Here's the drawing with two shaded views (mm, measured from the low corner). I have some questions. Round coordinates to 2 decimals unless told otherwise and drop trailing zeros. Loops run counter-clockwise (first coordinate to the right, second up) from the corner with the lowest first, then second, coordinate; pieces in that order, holes last. Notation, with made-up numbers: (72, 7) - (89, 7) arc R23 cw to (89, 34) - close; hole circle Ø8 at (-3, 52.5). An arc over 180 degrees is marked (long way). Use one line per item in the form item = value.
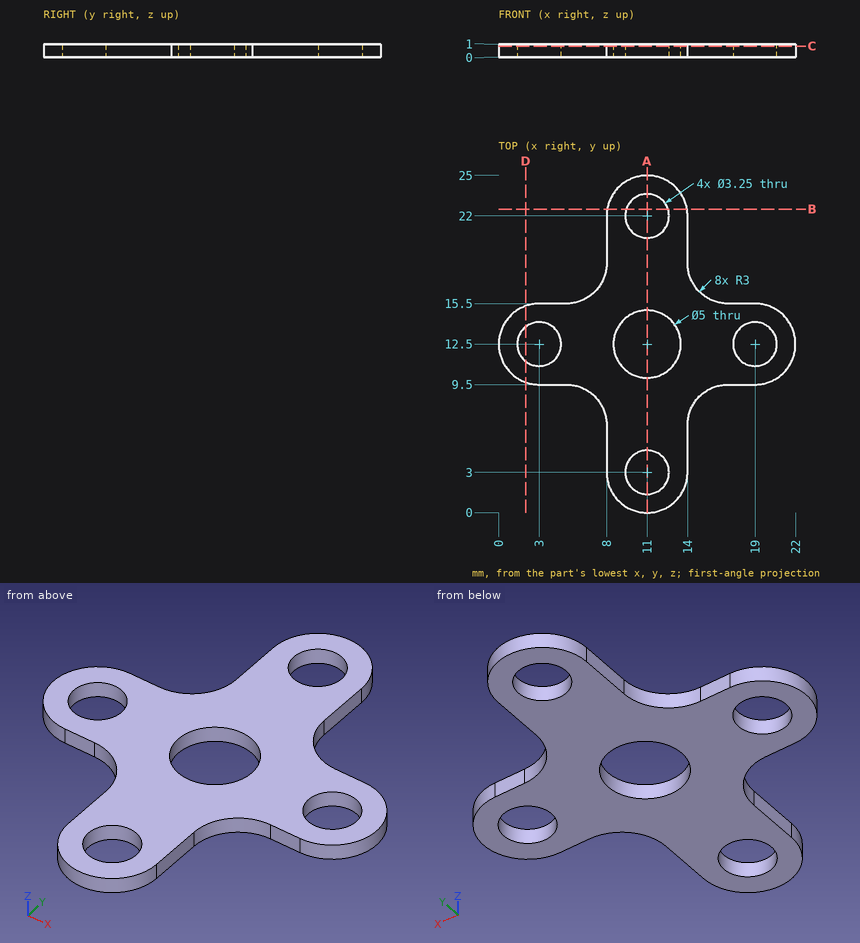
1. If we section it at A-A, the plane x = 11: Write out the boundary of the cut face in (y, z) (3 decimals), plus the area to 3 significant figures.
Solution:
outline = (0, 0) - (1.375, 0) - (1.375, 1) - (0, 1) - close; (4.625, 0) - (10, 0) - (10, 1) - (4.625, 1) - close; (15, 0) - (20.375, 0) - (20.375, 1) - (15, 1) - close; (23.625, 0) - (25, 0) - (25, 1) - (23.625, 1) - close
area = 13.5 mm^2
2. If we section it at B-B, the plane y = 22.5: Write out the boundary of the cut face in (x, z).
Solution:
outline = (8.04, 0) - (9.45, 0) - (9.45, 1) - (8.04, 1) - close; (12.55, 0) - (13.96, 0) - (13.96, 1) - (12.55, 1) - close
3. For P1, Ø5, axis at x = 11, y = 22, coming from the -Z side; P2, Ø3, axis at x = 19, y = 12.5, coming from the -Z side; P3, Ø0.5, axis at y = 5, z = 0.5, coming from the -X side; P4, Ø0.5, axis at x = 17.5, z = 0.5, coming from the +Y side, each with a flat end and sliding along its axis, tell me the tip position at first contact or that it passes through.
Solution:
P1 = 0
P2 = through
P3 = 8
P4 = 15.5
4. Please list where these lines run through material, in increasing order: line 1 along Y through (x, z) = (11, 0.55) (3 decimals); line 2 along Y through (x, z) = (3, 0.7) (3 decimals); line 3 along X through (y, z) = (20, 0.35).
Solution:
line_1 = 0 to 1.375, 4.625 to 10, 15 to 20.375, 23.625 to 25
line_2 = 9.5 to 10.875, 14.125 to 15.5
line_3 = 8 to 14
5. If we section it at C-C, the plane z = 0.85: Write out the boundary of the cut face in (x, y) (3 decimals).
Solution:
outline = (3, 9.5) - (5, 9.5) arc R3 cw to (8, 6.5) - (8, 3) arc R3 ccw to (14, 3) - (14, 6.5) arc R3 cw to (17, 9.5) - (19, 9.5) arc R3 ccw to (19, 15.5) - (17, 15.5) arc R3 cw to (14, 18.5) - (14, 22) arc R3 ccw to (8, 22) - (8, 18.5) arc R3 cw to (5, 15.5) - (3, 15.5) arc R3 ccw to start; hole circle Ø3.25 at (3, 12.5); hole circle Ø5 at (11, 12.5); hole circle Ø3.25 at (11, 3); hole circle Ø3.25 at (11, 22); hole circle Ø3.25 at (19, 12.5)
6. If we section it at D-D, the plane x = 2: Write out the boundary of the cut face in (y, z).
Solution:
outline = (9.67, 0) - (11.22, 0) - (11.22, 1) - (9.67, 1) - close; (13.78, 0) - (15.33, 0) - (15.33, 1) - (13.78, 1) - close
